Verification items for the finished model (mm, model axes). A direction names the side the tool comes from. Round coordinates to 2 decimals unless told otherwise and drop trailing zeros. Order: outer loops, then holes, each group sorted by start corner. A loop starts at its lowest first (then second) coordinate and runs counter-clockwise, first axis right, second up. Notation, with made-up numbers: (18.5, -25) -> (58.5, -25) arc R6 ccw to (58.5, -16) -> close; hole circle Ø4 at (8.5, 3.5). An arc over 180 degrees is marked (long way). Answer in a Markdown table with one row per item. Add a question column.
```python
from build123d import *

# Parameters (mm, degrees)
F0_W     = 254
F0_H     = 1155.7
F1_DEPTH = 3.175
F2_W     = 3.175
F2_H     = 1155.7
F3_DEPTH = 76.2
F4_W     = 3.175
F4_H     = 1155.7
F5_DEPTH = 101.6


with BuildPart() as f1:
    # F0 (on Top) → F1 (new body)
    with BuildSketch(Plane.XY):
        with Locations((127, 577.85)):
            Rectangle(F0_W, F0_H)
    extrude(amount=F1_DEPTH)

    # F2 (on face) → F3 (join)
    with BuildSketch(Plane.XY.offset(3.175)):
        with Locations((1.5875, 577.85)):
            Rectangle(F2_W, F2_H)
    extrude(amount=F3_DEPTH)

    # F4 (on face) → F5 (join)
    with BuildSketch(Plane(origin=(0, 0, 0), x_dir=(1, 0, 0), z_dir=(0, 0, -1))):
        with Locations((252.4125, -577.85)):
            Rectangle(F4_W, F4_H)
    extrude(amount=F5_DEPTH)


solid = f1.part
```
1) Cross-section at C-C, the plane x = 35. Record the boundary of the cut face in (y, z) (3 decimals).
2) Cross-section at A-A, the plane y = 625. Record the boundary of the cut face in (x, z) (3 decimals).
3) Depth check by flat-ended pin: P1, Ø1, axis at x = 129.5, y = 541, coming from the +Z side (3 decimals); P2, Ø1.5, axis at x = 225, y = 218, coming from the -Z side; P3, Ø1, axis at y = 445, z = 54.5, coming from the +X side (3 decimals). Enter the tip coordinate at first touch or a pass-through.
4) Cross-section at B-B, the plane z = -70.5. Record the boundary of the cut face in (x, y) (3 decimals).
5) Tool access check on faces 1 (the face through (254, 586, -48)), 2 (the face through (3.175, 570, 41)), 3 (the face through (124, 586, 0)). Record the directions out of +Z, -Z, +X, -X, +Y, -Y that give a thin tool (end or side, any length) a straight path to the whole face; none if there is none.
6) Thickness scan on L1, parallel to X at y = 105, z = -37.5 (3 decimals); L2, parallel to Z at x = 16, y = 320 (3 decimals). Record the ranges inside material, lowest first. Write a range as [from, to].
Results below:
| question | item | result |
|---|---|---|
| 1 | outline | (0, 0) -> (1155.7, 0) -> (1155.7, 3.175) -> (0, 3.175) -> close |
| 2 | outline | (0, 0) -> (250.825, 0) -> (250.825, -101.6) -> (254, -101.6) -> (254, 3.175) -> (3.175, 3.175) -> (3.175, 79.375) -> (0, 79.375) -> close |
| 3 | P1 | z = 3.175 |
| 3 | P2 | z = 0 |
| 3 | P3 | x = 3.175 |
| 4 | outline | (250.825, 0) -> (254, 0) -> (254, 1155.7) -> (250.825, 1155.7) -> close |
| 5 | face 1 | +Z, -Z, +X, +Y, -Y |
| 5 | face 2 | +Z, +X, +Y, -Y |
| 5 | face 3 | -Z, -X, +Y, -Y |
| 6 | L1 | [250.825, 254] |
| 6 | L2 | [0, 3.175] |
